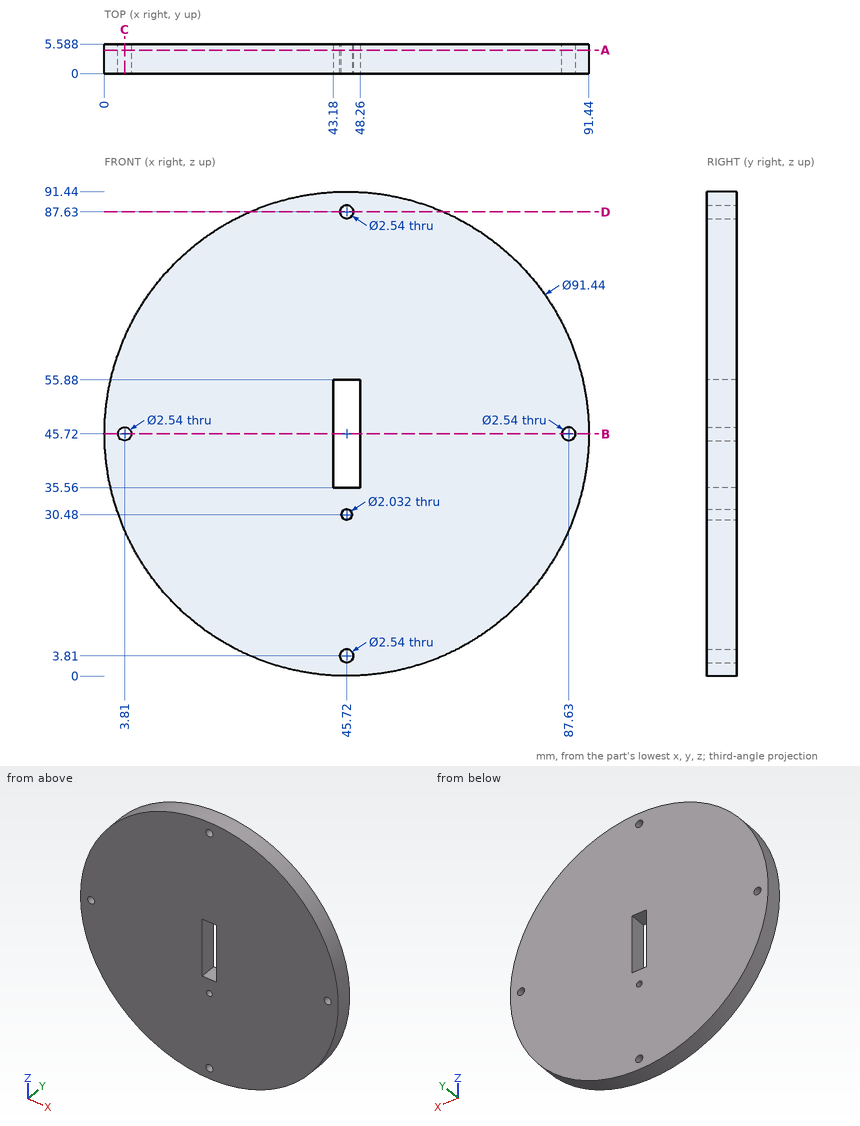
Geometry: see drawing. Coordinates: mm, zero at the bounding-box minimum. Give positions to 0.01 mm unless a question says otherwise; leave off trailing zeros. Write each loop counter-clockwise with the first axis right and the second up, starting at its lowest first coordinate (ties: lowest second). Pieces come first, ordered by that corner, then holes. Notation, with made-up numbers: M 10.25,-11.5 L 67.25,-11.5 A11 cw 67.25,8.5 Z; hole C -32,74.5 d8. An arc over 180 degrees is marked long. Answer as a JSON object with one key per item and string values.
Q1. Cut plane C-C, the plane x = 3.81. Return the cut outline in (y, z), then the cut area to 3 significant figures.
Geometry check:
{"outline": "M 0,27.45 L 5.59,27.45 L 5.59,44.45 L 0,44.45 Z; M 0,46.99 L 5.59,46.99 L 5.59,63.99 L 0,63.99 Z", "area": "190 mm^2"}
Q2. Contact query for flat-ended pins moving along their axis: P1, Ø2, axis at x = 40.5, y = 4, coming from the +Z side; P2, Ø1.7, axis at y = 3, z = 44, coming from the -X side; P3, Ø1.5, axis at x = 46.5, y = 3.5, coming from the -Z side. Output: stop coordinate, or through.
Geometry check:
{"P1": "stops at z = 91.24", "P2": "stops at x = 0.01", "P3": "stops at z = 0"}
Q3. Cut plane A-A, the plane y = 4.45. Return the cut outline in (x, z), then the cut area to 3 significant figures.
Geometry check:
{"outline": "C 45.72,45.72 d91.44; hole C 3.81,45.72 d2.54; hole M 43.18,35.56 L 48.26,35.56 L 48.26,55.88 L 43.18,55.88 Z; hole C 45.72,3.81 d2.54; hole C 45.72,87.63 d2.54; hole C 45.72,30.48 d2.03; hole C 87.63,45.72 d2.54", "area": "6,440 mm^2"}
Q4. Cut plane B-B, the plane z = 45.72. Return the cut outline in (x, y), then the cut area to 3 significant figures.
Geometry check:
{"outline": "M 0,0 L 2.54,0 L 2.54,5.59 L 0,5.59 Z; M 5.08,0 L 43.18,0 L 43.18,5.59 L 5.08,5.59 Z; M 48.26,0 L 86.36,0 L 86.36,5.59 L 48.26,5.59 Z; M 88.9,0 L 91.44,0 L 91.44,5.59 L 88.9,5.59 Z", "area": "454 mm^2"}
Q5. Cut plane D-D, the plane z = 87.63. Return the cut outline in (x, y).
Geometry check:
{"outline": "M 27.45,0 L 44.45,0 L 44.45,5.59 L 27.45,5.59 Z; M 46.99,0 L 63.99,0 L 63.99,5.59 L 46.99,5.59 Z"}
Q6. Ray query, line 1 along Z through (x, y) = (45.72, 2.9); line 2 along X through (y, z) = (1.1, 46); line 3 along X through (y, z) = (1.8, 87.63). Return the intervals inside material, ascending.
Geometry check:
{"line 1": "z = 0 to 2.54, 5.08 to 29.46, 31.5 to 35.56, 55.88 to 86.36, 88.9 to 91.44", "line 2": "x = 0 to 2.57, 5.05 to 43.18, 48.26 to 86.39, 88.87 to 91.44", "line 3": "x = 27.45 to 44.45, 46.99 to 63.99"}
